from build123d import *

# Parameters (mm, degrees)
CUT_EXTRUDE3_START = -28.048647
CUT_EXTRUDE3_DEPTH = 25.508647
CIRPATTERN2_COUNT  = 8
CUT_EXTRUDE4_REACH = 31.45
SKETCH6_R          = 12.59210321
SCALE1_SCALE       = 0.96551724


with BuildPart() as part:
    # Sketch1 → Revolve1 (revolve)
    with BuildSketch(Plane.XY, mode=Mode.PRIVATE) as revolve1_sk:
        with BuildLine():
            Line((-92.075, 0), (-92.075, -5.649667396))
            Line((-92.075, -5.649667396), (-67.31, -5.649667396))
            Line((-67.31, -5.649667396), (-67.31, -29.740701954))
            Line((-67.31, -29.740701954), (0, -29.740701954))
            Line((0, -29.740701954), (0, 0))
            Line((0, 0), (0, 23.771242064))
            ThreePointArc((0, 23.771242064), (-47.656193975, 18.155434253), (-92.075, 0))
        make_face()
    revolve(revolve1_sk.sketch.rotate(Axis((0, 46.369911649, 0), (0, -1, 0)), 270), axis=Axis((0, 46.369911649, 0), (0, -1, 0)))  # turned: the seam where the file's is

    # Sketch4 → Cut-Extrude3 (cut)
    with BuildSketch(Plane.XZ.offset(5.649667396).offset(CUT_EXTRUDE3_START)):
        with BuildLine():
            Line((24.987766053, 5.028443659), (74.822826668, 15.057063026))
            ThreePointArc((74.822826668, 15.057063026), (76.318746359, -0.787077909), (74.496377234, -16.596997215))
            Line((74.496377234, -16.596997215), (24.878745284, -5.542718741))
            ThreePointArc((24.878745284, -5.542718741), (25.487342091, -0.262851853), (24.987766053, 5.028443659))
        make_face()
    cut_extrude3 = extrude(amount=CUT_EXTRUDE3_DEPTH, mode=Mode.SUBTRACT)

    # CirPattern2: Cut-Extrude3 ×8 about axis
    cirpattern2_axis = Axis((0, 0, 0), (0, 1, 0))
    for i in range(1, CIRPATTERN2_COUNT):
        add(cut_extrude3.rotate(cirpattern2_axis, i * 360 / CIRPATTERN2_COUNT), mode=Mode.SUBTRACT)

    # Sketch6 → Cut-Extrude4 (cut, up to next)
    with BuildSketch(Plane.XZ.offset(5.649667396), mode=Mode.PRIVATE) as cut_extrude4_sk1:
        with Locations(Location((0, 0, 0), (0, 0, 270))):  # turned: the seam where the file's is
            Circle(SKETCH6_R)
    cut_extrude4_tool1 = extrude(cut_extrude4_sk1.sketch, amount=-CUT_EXTRUDE4_REACH, mode=Mode.PRIVATE) & part.part
    add(cut_extrude4_tool1.solids().sort_by_distance((0, -5.649667, 0))[0], mode=Mode.SUBTRACT)


with BuildPart() as part_1:
    # Scale1: scaled about (-5e-09, -7.646574392, 0)
    add(part.part.scale(SCALE1_SCALE).moved(Location((0, -0.26367499, 0))))


solid = part_1.part
Here's how the part is built. I have some questions about the finished solid (model axes, mm). A direction names the side the tool comes from. Give positions to 0.01 mm unless a question says otherwise; leave off trailing zeros. Loops run counter-clockwise (first coordinate to the right, second up) from the corner with the lowest first, then second, coordinate; pieces in that order, holes last. Notation, with made-up numbers: (48, -35) -> (63, -35) arc R27 ccw to (63, -17) -> close; hole circle Ø9 at (78.5, 54). An arc over 180 degrees is marked (long way). Answer as a JSON object with one key per item and string values. Group by question number.
Item 1: Imagine slicing it at A-A on y = -14.5. Write out the boundary of the cut face in (x, z).
Item 2: Will these pins go through, and if not, where does the flat tip stop? pin 1 (1 mm diameter, centred on x = -39.5, y = -9.5, fed in from +Z); pin 2 (1.5 mm diameter, centred on y = -22, z = -29.5, fed in from +X); pin 3 (7.5 mm diameter, centred on x = -1, z = 4.5, fed in from +Y).
Item 3: I need wall thicknesses on L1, parallel to X at y = 9.75, z = 0; L2, parallel to Y at x = 61, z = -5; L3, parallel to X at y = 2, z = 0. Which ranges of each line are inside material? Lowest first, please.
Item 4: On a 3-axis mill with a long thin cutter (end or side, diameter ignored), from which of +Z, -Z, +X, -X, +Y, -Y can I reach the whole of each face in a straight line? I mean faces 1 (the flat face through (65, -5.719, 6)), 2 (the flat face through (-8.553, 6.484, 42.501)). Say none if no direction works.
Item 5: Thinking about a two-plate mould opening in X: for faces 3 (the flat face through (-42.987, 6.484, 9.577)), 4 (the cylindrical face through (-74.96, -3.03, 47.79)), 5 (the flat face through (-1, -28.979, -1)), which applies, pulls with the +X half, pulls with the -X half, needs draft (parallel to the pull), parting line crosses it, or undercut?
Answer list:
{
 "1": {"outline": "circle Ø129.98 at (0, 0)"},
 "2": {"pin 1": "stops at z = 51.99", "pin 2": "stops at x = 58.28", "pin 3": "stops at y = -5.72"},
 "3": {"L1": "x = -24.61 to -12.16, 12.16 to 24.61", "L2": "y = -28.98 to -3.27", "L3": "x = -84.85 to -73.69, -24.61 to -12.16, 12.16 to 24.61, 73.69 to 84.85"},
 "4": {"face 1": "-Y", "face 2": "+Y"},
 "5": {"face 3": "undercut", "face 4": "parting line crosses it", "face 5": "needs draft"}
}
